Design review of the part built by this model. Coordinates are the model's own, in mm. A direction names the side the tool comes from. Coordinates: 2 decimals unless noted, no trailing zeros. Answer as a JSON object with one key per item and string values.
Autodesk Inventor part; units mm, degrees
ref_plane "РабПлоскость1" through (0, 34, 0) normal (0, 1, 0) x (-1, 0, 0)
ref_plane "YZ Plane" through (0, 0, 0) normal (1, 0, 0) x (0, 1, 0)
ref_plane "XY Plane" through (0, 0, 0) normal (0, 0, 1) x (1, 0, 0)
sketch "Эскиз1" plane through (0, 0, 0) normal (0, 0, 1) x (1, 0, 0)
  circle A0 centre (0, 0) radius 34
  dimension "d0" = 68
extrude "Выдавливание1" add sketch "Эскиз1" along normal mid plane 10
sketch "Эскиз2" plane through (0, 0, 5) normal (0, 0, 1) x (1, 0, 0)
  point P0 (0, 0)
  point P1 (0, 0)
hole "Отверстие1" at (0, 0, 5) direction (0, 0, -1) diameter 46.376 end through all
ref_plane "РабПлоскость1" through (0, 34, 0) normal (0, 1, 0) x (-1, 0, 0)
sketch "Эскиз3" plane through (0, 34, 0) normal (0, 1, 0) x (-1, 0, 0)
  point P0 (0, 0)
hole "Отверстие2" at (0, 34, 0) direction (0, -1, 0) diameter 6 depth 5 tip angle 118
pattern_circular "Круговой массив1" count 4 over 360 about axis through (0, 0, 0) along (0, 0, 1) of "Отверстие2"
chamfer "Фаска1" distance 1 angle 45 4 edges at (0, 23.188, 5) (0, 23.188, -5) (-34, 0, 5) (-34, 0, -5)
properties part number "05.01.002" material "Сталь, углеродистая"
(1) To check wall thickness, follow line 1 (Z direction, x = -31, y = 0); line 2 (Y direction, x = 0, z = 1.75); line 3 (Y direction, x = -18, z = -1.5). State the ranges of each line that lie inside material, in increasing order. Write a range as from..to.
Solved:
{"line 1": "z = -5..-3, 3..5", "line 2": "y = -28.25..-23.19, 23.19..28.25", "line 3": "y = -28.84..-14.62, 14.62..28.84"}
(2) Tool access review of faces 1 (the face through (-3, 31, 0)), 2 (the face through (0.9, -31.47, 2.86)), 3 (the face through (31, 0, -3)): name each direction out of +Z, -Z, +X, -X, +Y, -Y from which nothing blocks a thin tool from reaching the whole face with its end or side.
Solved:
{"face 1": "+Y", "face 2": "-Y", "face 3": "+X"}
(3) For pin 1 (1.5 mm diameter, centred on x = -22.5, z = 3.5, fed in from +Y); pin 2 (5 mm diameter, centred on x = 12, z = 1, fed in from +Y); pin 3 (3.5 mm diameter, centred on x = 0, z = 0, fed in from -Y), all flat-tipped, find the tip position at first contact; note any pin that passes through.
Solved:
{"pin 1": "stops at y = 26.13", "pin 2": "stops at y = 32.65", "pin 3": "stops at y = -28.25"}
(4) The part is to be moulded in two halves that separate along Y. For faces 4 (the face through (32.43, -10.21, -0.06)), 5 (the face through (-17.3, 17.3, 5)), 6 (the face through (-31.47, -0.9, 2.86)), 7 (the face through (27.51, -0.156, 0.497)), say which applies: pulls with the +Y half, pulls with the -Y half, needs draft (parallel to the pull), parting line crosses it, or undercut.
Solved:
{"face 4": "parting line crosses it", "face 5": "needs draft", "face 6": "undercut", "face 7": "undercut"}
